```python
from build123d import *

# Parameters (mm, degrees)
ESCALERA_DEPTH             = 37.5
CROQUIS_AGUJEROS_MONTAJE_R = 4
AGUJERO_INSERTO_M6_DEPTH   = 14


with BuildPart() as part:
    # Croquis_perfil_escalera → Escalera (new, symmetric)
    with BuildSketch(Plane.XY):
        Polygon((-87.5, 0), (87.5, 0), (87.5, 120), (12.5, 120), (12.5, 80), (-37.5, 80), (-37.5, 40), (-87.5, 40), align=None)
    extrude(amount=ESCALERA_DEPTH, both=True)

    # Croquis_agujeros_montaje → Agujero_inserto_M6 (cut)
    with BuildSketch(Plane(origin=(0, 0, 0), x_dir=(1, 0, 0), z_dir=(0, 1, 0))):
        with Locations(Location((-50, 0, 0), (0, 0, 270))):
            Circle(CROQUIS_AGUJEROS_MONTAJE_R)
        with Locations(Location((50, 0, 0), (0, 0, 270))):
            Circle(CROQUIS_AGUJEROS_MONTAJE_R)
    extrude(amount=AGUJERO_INSERTO_M6_DEPTH, mode=Mode.SUBTRACT)


solid = part.part
```
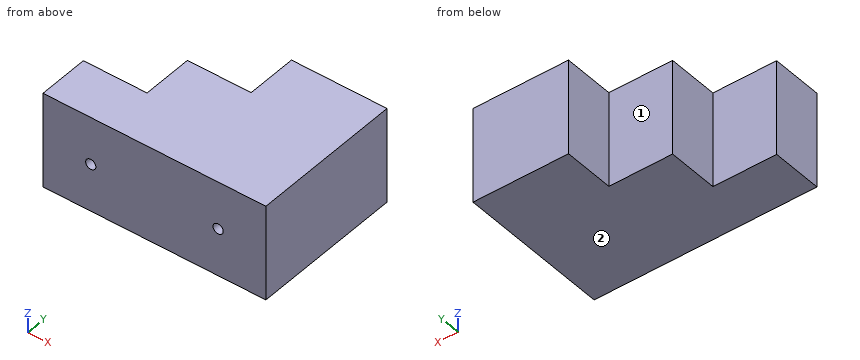
For this review, take the finished solid that the model builds, in its own axes (mm). Face numbers are marked on the shaded views. A direction names the side the tool comes from. Coordinates: 2 decimals unless noted, no trailing zeros. Loops run counter-clockwise (first coordinate to the right, second up) from the corner with the lowest first, then second, coordinate; pieces in that order, holes last.
1. Add section A-A, the plane z = 15. Give the boundary of the cut face in (x, y).
2. For the marked faces 1 and 2, list the 3-axis set-ups (+Z, -Z, +X, -X, +Y, -Y) from which the entire face can be reached by the end or side of a thin tool; tool diameter is ignored.
3. Insertion check: P1, Ø9, axis at x = -50.5, z = 1.5, coming from the -Y side; P2, Ø5, axis at x = -50, z = 0, coming from the -Y side; P3, Ø15, axis at x = -60, z = 11.5, coming from the +Y side; P4, Ø12, axis at y = 60.5, z = -4.5, coming from the -X side. Each pin has a flat end and moves straight along its axis. Give the tip position at first contact, or say it passes through.
4. Add section C-C, the plane y = 83. Give the boundary of the cut face in (x, z).
5. Add section D-D, the plane z = 0. Give the boundary of the cut face in (x, y), then the cut area to 3 significant figures.
6. For line 1 (X direction, y = 7.5, z = 0); line 2 (X direction, y = 84.5, z = 4); line 3 (Y direction, x = -64, z = -19), list the stretches that pass through material, from the lowest coordinate up.
7. Add section B-B, the plane x = -42.5. Give the boundary of the cut face in (y, z), then the cut area to 3 significant figures.
Result:
1. outline: (-87.5, 0) - (87.5, 0) - (87.5, 120) - (12.5, 120) - (12.5, 80) - (-37.5, 80) - (-37.5, 40) - (-87.5, 40) - close
2. face 1: +Z, -Z, -X, +Y
2. face 2: -Z, +X, -X, +Y, -Y
3. P1: stops at y = 0
3. P2: stops at y = 14
3. P3: stops at y = 40
3. P4: stops at x = -37.5
4. outline: (12.5, -37.5) - (87.5, -37.5) - (87.5, 37.5) - (12.5, 37.5) - close
5. outline: (-87.5, 0) - (-54, 0) - (-54, 14) - (-46, 14) - (-46, 0) - (46, 0) - (46, 14) - (54, 14) - (54, 0) - (87.5, 0) - (87.5, 120) - (12.5, 120) - (12.5, 80) - (-37.5, 80) - (-37.5, 40) - (-87.5, 40) - close
5. area: 14,800 mm2
6. line 1: x = -87.5 to -54, -46 to 46, 54 to 87.5
6. line 2: x = 12.5 to 87.5
6. line 3: y = 0 to 40
7. outline: (0, -37.5) - (40, -37.5) - (40, 37.5) - (0, 37.5) - close
7. area: 3,000 mm2
